Autodesk Inventor part; units mm, degrees
ref_plane "YZ Plane" through (0, 0, 0) normal (1, 0, 0) x (0, 1, 0)
ref_plane "XZ Plane" through (0, 0, 0) normal (0, 1, 0) x (-1, 0, 0)
ref_plane "XY Plane" through (0, 0, 0) normal (0, 0, 1) x (1, 0, 0)
sketch "Sketch1" plane through (0, 0, 0) normal (0, 0, 1) x (1, 0, 0)
  line L0 (76.176, -10.7873) -> (76.176, 14.6127)
  line L1 (-76.176, 10.7873) -> (-76.176, -14.6127)
  line L2 (-76.176, -14.6127) -> (76.176, 14.6127) construction
  line L3 (76.176, -10.7873) -> (-76.176, 10.7873) construction
  line L4 (76.176, 9.4269) -> (81.6753, -0.0981)
  line L5 (81.6753, -0.0981) -> (76.176, -9.6231)
  line L6 (76.176, -9.6231) -> (65.1775, -9.6231)
  line L7 (65.1775, -9.6231) -> (59.6782, -0.0981)
  line L8 (59.6782, -0.0981) -> (65.1775, 9.4269)
  line L9 (65.1775, 9.4269) -> (76.176, 9.4269)
  line L10 (76.176, 9.4269) -> (76.176, -9.6231) construction
  line L11 (-54.9157, 9.1213) -> (-49.4164, -0.4037)
  line L12 (-49.4164, -0.4037) -> (-54.9157, -9.9287)
  line L13 (-54.9157, -9.9287) -> (-65.9142, -9.9287)
  line L14 (-65.9142, -9.9287) -> (-71.4135, -0.4037)
  line L15 (-71.4135, -0.4037) -> (-65.9142, 9.1213)
  line L16 (-65.9142, 9.1213) -> (-54.9157, 9.1213)
  line L17 (-76.176, -14.6127) -> (-38.076, -14.6127) construction
  line L18 (-38.076, -14.6127) -> (-38.076, 10.7873) construction
  line L19 (-40.1744, 10.7873) -> (-76.176, 10.7873) construction
  line L20 (-76.176, 10.7873) -> (-76.176, -14.6127) construction
  line L21 (76.176, 14.6127) -> (38.076, 14.6127) construction
  line L22 (38.076, 14.6127) -> (38.076, -10.7873) construction
  line L23 (38.076, -10.7873) -> (76.176, -10.7873) construction
  line L24 (76.176, -10.7873) -> (76.176, 14.6127) construction
  line L25 (-25.0148, -6.35) -> (25.0148, -6.35) construction
  line L26 (25.0148, -6.35) -> (25.0148, 6.35) construction
  line L27 (25.0148, 6.35) -> (-25.0148, 6.35) construction
  line L28 (-25.0148, 6.35) -> (-25.0148, -6.35) construction
  line L29 (-25.0148, -6.35) -> (25.0148, 6.35) construction
  line L30 (25.0148, -6.35) -> (-25.0148, 6.35) construction
  line L31 (-36.0891, 10.1123) -> (-25.0148, 6.35)
  line L32 (25.0148, 6.35) -> (38.076, 14.6127)
  line L33 (25.0148, 6.35) -> (-25.0148, 6.35)
  line L34 (-38.076, -14.6127) -> (-25.0148, -6.35)
  line L35 (-25.0148, -6.35) -> (25.0148, -6.35)
  line L36 (25.0148, -6.35) -> (38.076, -10.7873)
  line L37 (76.176, 14.6127) -> (38.076, 14.6127)
  line L38 (-38.076, 10.7873) -> (-76.176, 10.7873)
  line L39 (-76.176, -14.6127) -> (-38.076, -14.6127)
  line L40 (38.076, -10.7873) -> (76.176, -10.7873)
  arc A0 (-36.0891, 10.1123) -> (-40.1744, 10.7873) centre (-40.1744, -1.9127) ccw
  point P0 (0, 0)
  point P1 (70.6767, -0.0981)
  point P2 (-60.415, -0.4037)
  point P3 (76.176, -9.6231)
  point P4 (76.176, 9.4269)
  dimension "totalLength" = 152.4
  dimension "d1" = 25.4
  dimension "d2" = 19.05
  dimension "d3" = 4.7625
  dimension "d4" = 19.05
  dimension "d5" = 38.1
  dimension "d6" = 38.1
  dimension "d8" = 12.7
  dimension "d9" = 12.7
extrude "Extrusion1" add sketch "Sketch1" along normal mid plane 6.35 contours L40 L36 L35 L34 L39 L1 L38 A0 L31 L33 L32 L37 L0 L9 L8 L7 L6
properties part number "Whack01"
Model file for the job. Use its own axes, mm. A direction names the side the tool comes from. Give positions to 0.01 mm unless a question says otherwise; leave off trailing zeros. Loops run counter-clockwise (first coordinate to the right, second up) from the corner with the lowest first, then second, coordinate; pieces in that order, holes last. Notation, with made-up numbers: M 34.5,-39 L 91.5,-39 A22 ccw 91.5,-5 Z; hole C 1,70.5 d5. An arc over 180 degrees is marked long. Use one line per item in the form item = value.
Item 1: Slice it at D-D on x = 21.5. List the corners of the cut face in (y, z) (3 decimals), and give its area (3 significant figures).
Filled in:
outline = M -6.35,-3.175 L 6.35,-3.175 L 6.35,3.175 L -6.35,3.175 Z
area = 80.6 mm^2
Item 2: Drill centre lines: L1, parallel to Y at x = 65.5, z = -1; L2, parallel to Y at x = 42, z = 2.75; L3, parallel to X at y = 5.5, z = -1.25. Where is each one in solid material? Low to high.
Filled in:
L1 = -10.79 to -9.62, 9.43 to 14.61
L2 = -10.79 to 14.61
L3 = -76.18 to -68, -52.82 to 62.91
Item 3: Two-plate mould, pull along X, no slides. Class faces 5 (the flat face through (-52.13, -5.1, -0.04)), 6 (the flat face through (71, 9.427, 0)), 7 (the flat face through (0, 6.35, 0)), 8 (the flat face through (-76.176, -2, 0)): released by +X, released by -X, zero draft, split by the parting line, or undercut.
Filled in:
face_5 = undercut
face_6 = zero draft
face_7 = undercut
face_8 = released by -X
Item 4: Slice it at C-C on y = -4.75. List the corners of the cut face in (x, z) (3 decimals), and give its area (3 significant figures).
Filled in:
outline = M -76.176,-3.175 L -68.904,-3.175 L -68.904,3.175 L -76.176,3.175 Z; M -51.926,-3.175 L 62.364,-3.175 L 62.364,3.175 L -51.926,3.175 Z
area = 772 mm^2
Item 5: Slice it at A-A on x = -61.5. List the corners of the cut face in (y, z) (3 decimals), and give its area (3 significant figures).
Filled in:
outline = M -14.613,-3.175 L -9.929,-3.175 L -9.929,3.175 L -14.613,3.175 Z; M 9.121,-3.175 L 10.787,-3.175 L 10.787,3.175 L 9.121,3.175 Z
area = 40.3 mm^2
Item 6: Slice it at B-B on z = -1.75. List the corners of the cut face in (x, y).
Filled in:
outline = M -76.18,-14.61 L -38.08,-14.61 L -25.01,-6.35 L 25.01,-6.35 L 38.08,-10.79 L 76.18,-10.79 L 76.18,-9.62 L 65.18,-9.62 L 59.68,-0.1 L 65.18,9.43 L 76.18,9.43 L 76.18,14.61 L 38.08,14.61 L 25.01,6.35 L -25.01,6.35 L -36.09,10.11 A12.7 ccw -40.17,10.79 L -76.18,10.79 Z; hole M -71.41,-0.4 L -65.91,-9.93 L -54.92,-9.93 L -49.42,-0.4 L -54.92,9.12 L -65.91,9.12 Z
Item 7: Which spindle directions (+Z, -Z, +X, -X, +Y, -Y) get a long thin tool onto all of the face, cutting with end or side? Do faces 1 (the flat face through (-60, 9.121, 0)), 2 (the cylindrical face through (-38.13, 10.62, -0.04)), 3 (the flat face through (31.454, -8.538, -0.044)), 4 (the flat face through (-58, 10.787, 0)). Say none if no direction does.
Filled in:
face_1 = +Z, -Z
face_2 = +Z, -Z, +Y
face_3 = +Z, -Z, -Y
face_4 = +Z, -Z, -X, +Y
Item 8: Flat gauge pins, fed straight in: pin 1 Ø3 at (x, z) = (-58.5, 1.5) entering from +Y; pin 2 Ø1 at (x, y) = (-29, 8.5) entering from +Z; pin 3 Ø3 at (x, z) = (51, -1) entering from -Y; pin 4 Ø1.9 at (x, z) = (4.5, -0.5) entering from +Y. Where does each tip first touch, or does it go through?
Filled in:
pin_1 = 10.79
pin_2 = through
pin_3 = -10.79
pin_4 = 6.35
